```python
from build123d import *

# Parameters (mm, degrees)
BOSS_EXTRUDE1_DEPTH     = 4.5
CUT_EXTRUDE1_DEPTH      = 77.442789065
CUT_EXTRUDE1_DEPTH_BACK = 77.442789065
SKETCH3_R               = 0.99
SKETCH4_R               = 5
CUT_EXTRUDE2_DEPTH      = 77.442789065
CUT_EXTRUDE3_DEPTH      = 77.442789065
CUT_EXTRUDE3_DEPTH_BACK = 77.442789065
SKETCH5_R               = 1.25
SKETCH5_R_2             = 5


with BuildPart() as part:
    # Sketch2 → Boss-Extrude1 (new, symmetric)
    with BuildSketch(Plane(origin=(0, 0, 0), x_dir=(1, 0, 0), z_dir=(0, 1, 0))):
        with BuildLine():
            Line((50, -22.5), (-50, -22.5))
            ThreePointArc((-50, -22.5), (-72.5, 0), (-50, 22.5))
            Line((-50, 22.5), (50, 22.5))
            ThreePointArc((50, 22.5), (72.5, 0), (50, -22.5))
        make_face()
    extrude(amount=BOSS_EXTRUDE1_DEPTH, both=True)

    # Sketch3 → Cut-Extrude1 (cut, two sides: drawn at the far end of the back side and taken through both)
    with BuildSketch(Plane(origin=(0, 4.5, 0), x_dir=(1, 0, 0), z_dir=(0, 1, 0)).offset(-CUT_EXTRUDE1_DEPTH_BACK)):
        with Locations(Location((41.95, 0, 0), (0, 0, 270))):
            Circle(SKETCH3_R)
        with Locations(Location((44.307790411, 5.692209589, 0), (0, 0, 270))):
            Circle(SKETCH3_R)
        with Locations(Location((50, 8.05, 0), (0, 0, 270))):
            Circle(SKETCH3_R)
        with Locations(Location((55.692209589, 5.692209589, 0), (0, 0, 270))):
            Circle(SKETCH3_R)
        with Locations(Location((58.05, 0, 0), (0, 0, 270))):
            Circle(SKETCH3_R)
        with Locations(Location((55.692209589, -5.692209589, 0), (0, 0, 270))):
            Circle(SKETCH3_R)
        with Locations(Location((50, -8.05, 0), (0, 0, 270))):
            Circle(SKETCH3_R)
        with Locations(Location((44.307790411, -5.692209589, 0), (0, 0, 270))):
            Circle(SKETCH3_R)
    extrude(amount=CUT_EXTRUDE1_DEPTH + CUT_EXTRUDE1_DEPTH_BACK, mode=Mode.SUBTRACT)

    # Sketch4 → Cut-Extrude2 (cut, through all)
    with BuildSketch(Plane(origin=(0, 4.5, 0), x_dir=(1, 0, 0), z_dir=(0, 1, 0))):
        with Locations(Location((50, 0, 0), (0, 0, 270))):
            Circle(SKETCH4_R)
    extrude(amount=-CUT_EXTRUDE2_DEPTH, mode=Mode.SUBTRACT)

    # Sketch5 → Cut-Extrude3 (cut, two sides: drawn at the far end of the back side and taken through both)
    with BuildSketch(Plane(origin=(0, 4.5, 0), x_dir=(1, 0, 0), z_dir=(0, 1, 0)).offset(-CUT_EXTRUDE3_DEPTH_BACK)):
        with Locations(Location((-51.5, -15.05, 0), (0, 0, 270))):
            Circle(SKETCH5_R)
        with Locations(Location((-51.5, 15.05, 0), (0, 0, 270))):
            Circle(SKETCH5_R)
        with Locations(Location((-11.1, 8.55, 0), (0, 0, 270))):
            Circle(SKETCH5_R)
        with Locations(Location((-11.1, -8.55, 0), (0, 0, 270))):
            Circle(SKETCH5_R)
        with Locations(Location((-47, 0, 0), (0, 0, 270))):
            Circle(SKETCH5_R_2)
    extrude(amount=CUT_EXTRUDE3_DEPTH + CUT_EXTRUDE3_DEPTH_BACK, mode=Mode.SUBTRACT)


solid = part.part
```
Geometry: final body of the model. Coordinates: model frame, mm. Give positions to 0.01 mm unless a question says otherwise; leave off trailing zeros. Loops run counter-clockwise (first coordinate to the right, second up) from the corner with the lowest first, then second, coordinate; pieces in that order, holes last. Notation, with made-up numbers: (27, -28) -> (33, -28) arc R12 cw to (33, -14) -> close; hole circle Ø7 at (48, 49). An arc over 180 degrees is marked (long way). Return JSON: item names as keys, results as strings.
Item 1: Section B-B, the plane y = -2.25. Count the separate pieces of the cut face and the enclosed holes in it, plus the area to 3 significant figures.
Filled in:
{"separate pieces": "1", "enclosed holes": "14", "area": "5,890 mm^2"}
Item 2: Mould query, pull axis Z, two halves, no side actions, for faces 1 (the flat face through (-1, 0, -22.5)), 2 (the cylindrical face through (54.957, 0.063, -0.651)), 3 (the flat face through (1, -4.5, 0)), 4 (the cylindrical face through (-72.495, 0.063, 0.495)). Classes: released by +Z, released by -Z, zero draft, split by the parting line, or undercut.
Filled in:
{"face 1": "released by -Z", "face 2": "undercut", "face 3": "zero draft", "face 4": "split by the parting line"}
Item 3: Line query: line 1 (Z direction, x = -47.5, y = 2.75); line 2 (Z direction, x = -50.5, y = 1); line 3 (X direction, y = 1, z = -8.05). Output: solid intervals per line, ascending.
Filled in:
{"line 1": "-22.5 to -4.97, 4.97 to 22.5", "line 2": "-22.49 to -15.8, -14.3 to -3.57, 3.57 to 14.3, 15.8 to 22.49", "line 3": "-71.01 to -12.25, -9.95 to 49.01, 50.99 to 71.01"}
Item 4: Pin query (flat end, axial travel): P1, Ø1, axis at y = 0.5, z = 17, coming from the -X side; P2, Ø2.5, axis at x = 55.69, z = -5.69, coming from the -Y side; P3, Ø4, axis at y = -3.5, z = 4, coming from the +X side; P4, Ø4, axis at y = 3, z = -15, coming from the +X side. Return the tip coordinate at first contact, or that it passes through.
Filled in:
{"P1": "x = -65.3", "P2": "y = -4.5", "P3": "x = 72.41", "P4": "x = 68.36"}
Item 5: Section C-C, the plane z = 15.05. Output: boundary loops of the cut face in (x, y), plus the area to 3 significant figures.
Filled in:
{"outline": "(-66.73, -4.5) -> (-52.75, -4.5) -> (-52.75, 4.5) -> (-66.73, 4.5) -> close; (-50.25, -4.5) -> (66.73, -4.5) -> (66.73, 4.5) -> (-50.25, 4.5) -> close", "area": "1,180 mm^2"}
Item 6: Section A-A, the plane x = -47. Output: boundary loops of the cut face in (y, z), plus the area to 3 significant figures.
Filled in:
{"outline": "(-4.5, -22.5) -> (4.5, -22.5) -> (4.5, -5) -> (-4.5, -5) -> close; (-4.5, 5) -> (4.5, 5) -> (4.5, 22.5) -> (-4.5, 22.5) -> close", "area": "315 mm^2"}
